CAD build for the part. Positions are in the model's coordinates, mm. A direction names the side the tool comes from. Round coordinates to 2 decimals unless told otherwise and drop trailing zeros. Loops run counter-clockwise (first coordinate to the right, second up) from the corner with the lowest first, then second, coordinate; pieces in that order, holes last. Notation, with made-up numbers: M 19,-21 L 24,-21 A36 cw 24,16 Z; hole C 23,-30.5 d10. An arc over 180 degrees is marked long. Use a Markdown table: item, result. Add a question column.
(1) Band-saw the part on D-D, the plane z = 94. Give the number of separate pieces and of enclosed holes in the cut face, and give its area (3 significant figures).
(2) Wall check: L1, parallel to Y at x = 21, z = -79; L2, parallel to Y at x = 2.5, z = 66.5; L3, parallel to Z at x = 10.5, y = -1. Give the ranges that are in metal, low to high.
(3) Band-saw the part on B-B, the plane z = -69. Write the cut outline in (x, y) (3 decimals).
(4) Flat gauge pins, fed straight in: P1, Ø12, axis at y = -43, z = 8.5, coming from the -X side; P2, Ø1.5, axis at x = 10, y = -36, coming from the +Z side; P3, Ø19, axis at y = 0.5, z = -112.5, coming from the -X side. Where does each tip first touch, or does it go through?
(5) Two-plate mould, pull along Z, no slides. Class faces 1 (the face through (0, 38, 2)), 2 (the face through (11, 25.4, -65)), 3 (the face through (11, 38, 77.788)): released by +Z, released by -Z, zero draft, split by the parting line, or undercut.
(6) Which spindle directions (+Z, -Z, +X, -X, +Y, -Y) get a long thin tool onto all of the face, cutting with end or side? Do faces 4 (the face through (11, -38, 77.788)), 5 (the face through (13, 0, -39.688)), 6 (the face through (2, -19.05, 46)). Say none if no direction does.
(7) Band-saw the part on A-A, the plane x = 19.75. Write the cut outline in (y, z), and give its area (3 significant figures).
from build123d import *

# Parameters (mm, degrees)
F0_W     = 114.3
F0_H     = 257.175
F0_W_2   = 50.8
F0_H_2   = 50.8
F1_DEPTH = 22.225
F2_W     = 4.7625
F2_H     = 38.1
F3_DEPTH = 257.176
F4_R     = 4.7625
F5_DEPTH = 50.8


with BuildPart() as f1:
    # F0 (on Right) → F1 (new body)
    with BuildSketch(Plane.YZ):
        Rectangle(F0_W, F0_H)
        with Locations((0, -65.0875)):
            Rectangle(F0_W_2, F0_H_2, mode=Mode.SUBTRACT)
    extrude(amount=F1_DEPTH)

    # F2 (on face) → F3 (cut, through all)
    with BuildSketch(Plane.XY.offset(128.5875)):
        with Locations((2.38125, 0)):
            Rectangle(F2_W, F2_H)
    extrude(amount=-F3_DEPTH, mode=Mode.SUBTRACT)

    # F4 (on face) → F5 (cut)
    with BuildSketch(Plane.XY.offset(128.5875)):
        with Locations((11.1125, -38.1)):
            Circle(F4_R)
        with Locations((11.1125, 38.1)):
            Circle(F4_R)
    extrude(amount=-F5_DEPTH, mode=Mode.SUBTRACT)


solid = f1.part
Return value:
| question | item | result |
|---|---|---|
| 1 | separate pieces | 1 |
| 1 | enclosed holes | 2 |
| 1 | area | 2,220 mm^2 |
| 2 | L1 | -57.15 to -25.4, 25.4 to 57.15 |
| 2 | L2 | -57.15 to -19.05, 19.05 to 57.15 |
| 2 | L3 | -128.59 to -90.49, -39.69 to 128.59 |
| 3 | outline | M 0,-57.15 L 22.225,-57.15 L 22.225,-25.4 L 0,-25.4 Z; M 0,25.4 L 22.225,25.4 L 22.225,57.15 L 0,57.15 Z |
| 4 | P1 | x = 0 |
| 4 | P2 | z = 77.79 |
| 4 | P3 | x = 4.76 |
| 5 | face 1 | zero draft |
| 5 | face 2 | undercut |
| 5 | face 3 | released by +Z |
| 6 | face 4 | +Z |
| 6 | face 5 | +X, -X |
| 6 | face 6 | +Z, -Z, -X |
| 7 | outline | M -57.15,-128.59 L 57.15,-128.59 L 57.15,128.59 L -57.15,128.59 Z; hole M -25.4,-90.49 L 25.4,-90.49 L 25.4,-39.69 L -25.4,-39.69 Z |
| 7 | area | 26,800 mm^2 |
